Could you check a few things on this drawing? It's one solid part, dimensions in mm from its lowest x, y, z. Coordinates: 2 decimals unless noted, no trailing zeros. Order: outer loops, then holes, each group sorted by start corner. A loop starts at its lowest first (then second) coordinate and runs counter-clockwise, first axis right, second up. Notation, with made-up numbers: (-12, 3.25) - (12, 3.25) arc R22 cw to (12, 27.25) - close; hole circle Ø8 at (7, 69). An arc over 180 degrees is marked (long way). Return JSON: item names as keys, results as strings. Group by question number.
1) Imagine slicing it at D-D (x = 40). Write out the boundary of the cut face in (y, z).
2) If I drill on line 1 along X through (y, z) = (1.8, 22.5); line 2 along Z through (x, y) = (22.5, 7.05); line 3 along Y through (x, z) = (30, 14), over which ranges is the centre line in solid material (lowest first)?
3) Imagine slicing it at A-A (z = 22.5). Write out the boundary of the cut face in (x, y), and give its area (3 significant figures).
4) For pin 1 Ø2 at (x, y) = (15, 7) entering from -Z; pin 2 Ø16.5 at (x, z) = (17.5, 32.2) entering from +Y; pin 3 Ø1 at (x, z) = (12.5, 22.5) entering from -Y, each with a flat end and sliding along its axis, tell me the tip position at first contact or that it passes through.
5) Imagine slicing it at C-C (y = 7.75). Write out the boundary of the cut face in (x, z).
6) Imagine slicing it at B-B (x = 29.5). Write out the boundary of the cut face in (y, z).
7) If we mould it in two halves opening along Z, with no side actions, what happens to the marked faces 1, 2, 3 and 4? For each: pulls with the +Z half, pulls with the -Z half, needs draft (parallel to the pull), parting line crosses it, or undercut.
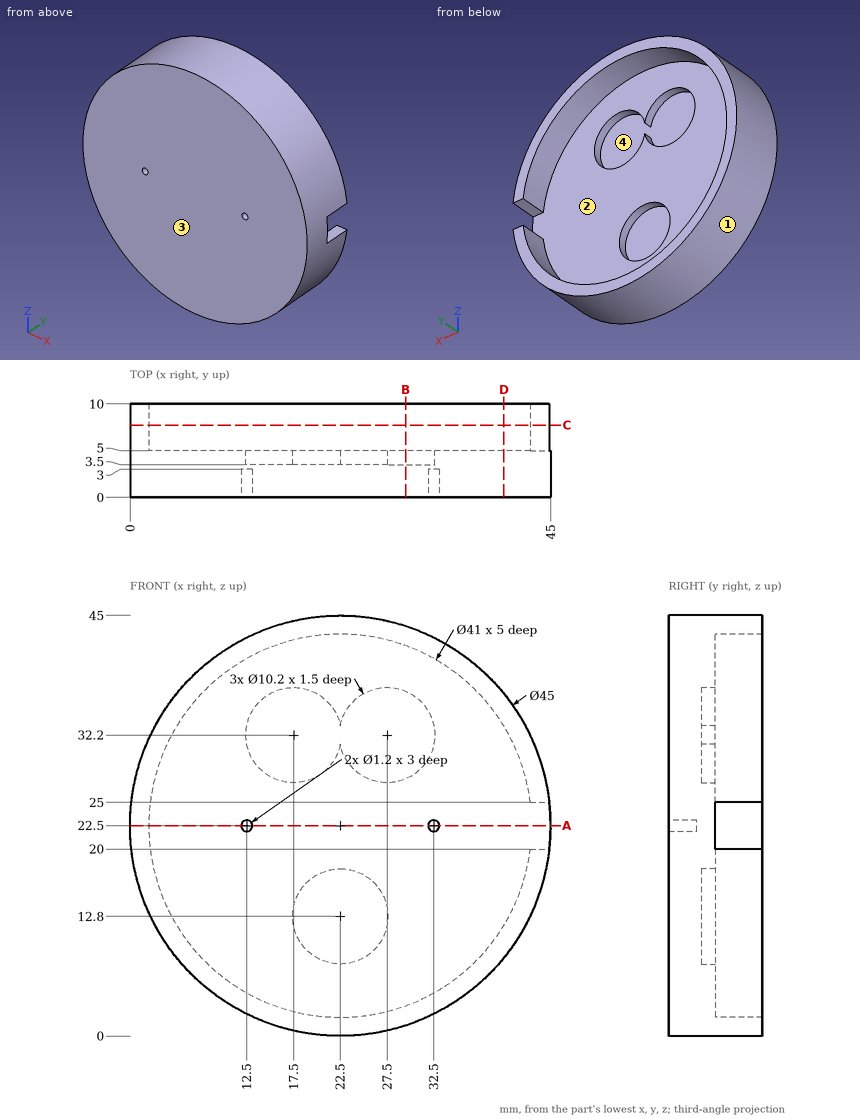
Calculated:
{
 "1": {"outline": "(0, 8.36) - (10, 8.36) - (10, 11.82) - (5, 11.82) - (5, 33.18) - (10, 33.18) - (10, 36.64) - (0, 36.64) - close"},
 "2": {"line 1": "0 to 11.9, 13.1 to 31.9, 33.1 to 45", "line 2": "0 to 2, 43 to 45", "line 3": "0 to 5"},
 "3": {"outline": "(0, 0) - (11.9, 0) - (11.9, 3) - (13.1, 3) - (13.1, 0) - (31.9, 0) - (31.9, 3) - (33.1, 3) - (33.1, 0) - (45, 0) - (45, 5) - (2, 5) - (2, 10) - (0, 10) - close", "area": "228 mm2"},
 "4": {"pin 1": "z = 0.96", "pin 2": "y = 5", "pin 3": "y = 3"},
 "5": {"outline": "(42.85, 20) arc R20.5 cw (long way) to (42.85, 25) - (44.86, 25) arc R22.5 ccw (long way) to (44.86, 20) - close"},
 "6": {"outline": "(0, 1.12) - (10, 1.12) - (10, 3.23) - (5, 3.23) - (5, 27.51) - (3.5, 27.51) - (3.5, 36.89) - (5, 36.89) - (5, 41.77) - (10, 41.77) - (10, 43.88) - (0, 43.88) - close"},
 "7": {"face 1": "parting line crosses it", "face 2": "undercut", "face 3": "needs draft", "face 4": "undercut"}
}
